Design review of the part built by this model. Coordinates are the model's own, in mm. A direction names the side the tool comes from. Coordinates: 2 decimals unless noted, no trailing zeros. Loops run counter-clockwise (first coordinate to the right, second up) from the corner with the lowest first, then second, coordinate; pieces in that order, holes last. Notation, with made-up numbers: M 14.25,39 L 45.25,39 A26 ccw 45.25,63 Z; hole C 88.25,-7 d11. An arc over 180 degrees is marked long. Answer as a JSON object with one key per item and string values. Group by question number.
1. Consider section B-B (y = 10.9). State the section outline as (x, z) points, then the cut area to 3 significant figures.
2. Machinability: for faces 4 (the flat face through (4, 20.2, 5)), 5 (the flat face through (8, 21, 5)), 6 (the flat face through (16, 0, 1)), which of the approach directions +Z, -Z, +X, -X, +Y, -Y give a long, thin tool a straight path to every point of the face, cutting with its end or side? Answer none if there is none.
3. Draft analysis for pull direction Y (two halves, no side actions). For faces 1 (the flat face through (0, 11, 1)), 2 (the flat face through (16, 21.8, 1)), 3 (the flat face through (4, 1.6, 5)), state which applies: +Y half, -Y half, draft (parallel to the pull), parting line (faces both ways), or undercut.
4. To check wall thickness, follow probe 1 along Y at (x, z) = (18, 0.5); probe 2 along Z at (x, y) = (48.5, 10.5); probe 3 along X at (y, z) = (10.5, 0.75). State the ranges of each line that lie inside material, in increasing order.
5. Consider section D-D (y = 3.5). State the section outline as (x, z) points.
6. Consider section A-A (z = 3). State the section outline as (x, y) points.
7. Insertion check: pin 1 (5 mm diameter, centred on y = 18.5, z = 10, fed in from +X); pin 2 (4 mm diameter, centred on x = 18, y = 10.9, fed in from +Z). Each pin has a flat end and moves straight along its axis. Give the tip position at first contact, or say it passes through.
8. Consider section C-C (x = 42). State the section outline as (y, z) points.
Autodesk Inventor part; units mm, degrees
ref_plane "YZ Plane" through (0, 0, 0) normal (1, 0, 0) x (0, 1, 0)
ref_plane "XZ Plane" through (0, 0, 0) normal (0, 1, 0) x (-1, 0, 0)
ref_plane "XY Plane" through (0, 0, 0) normal (0, 0, 1) x (1, 0, 0)
sketch "Sketch1" plane through (0, 0, 0) normal (0, 0, 1) x (1, 0, 0)
  line L0 (0, 0) -> (50, 0)
  line L1 (50, 0) -> (50, 21.8)
  line L2 (50, 21.8) -> (0, 21.8)
  line L3 (0, 21.8) -> (0, 0)
  circle A0 centre (42, 10.9) radius 1.65
  circle A1 centre (18, 10.9) radius 1.65
  dimension "d0" = 50
  dimension "d1" = 21.8
  dimension "d15" = 3.3
  dimension "d16" = 3.3
  dimension "d17" = 24
  dimension "d18" = 8
  dimension "d19" = 10.9
  dimension "d20" = 10.9
extrude "Extrusion1" add sketch "Sketch1" along normal blind 1.6
sketch "Sketch2" plane through (0, 0, 1.6) normal (0, 0, 1) x (1, 0, 0)
  line L0 (0, 21.8) -> (0, 0)
  line L1 (0, 0) -> (8, 0)
  line L2 (8, 0) -> (8, 1.6)
  line L3 (8, 1.6) -> (0, 1.6)
  line L4 (0, 1.6) -> (0, 0)
  line L5 (50, 21.8) -> (0, 21.8)
  line L6 (0, 21.8) -> (8, 21.8)
  line L7 (8, 21.8) -> (8, 20.2)
  line L8 (8, 20.2) -> (0, 20.2)
  line L9 (0, 20.2) -> (0, 21.8)
  point P0 (0, 20.2)
  dimension "d4" = 8
  dimension "d5" = 1.6
  dimension "d6" = 8
  dimension "d7" = 1.6
extrude "Extrusion2" add sketch "Sketch2" along normal blind 10
sketch "Sketch3" plane through (0, 0, 0) normal (0, -1, 0) x (1, 0, 0)
  circle A0 centre (4, 7.1) radius 1.65
  line L0 (0, 0) -> (0, 11.6)
  line L1 (0, 11.6) -> (8, 11.6)
  line L2 (0, 0) -> (50, 0)
  dimension "d10" = 3.3
  dimension "d11" = 4
  dimension "d21" = 7.1
extrude "Extrusion3" cut sketch "Sketch3" against normal blind 25
fillet "Fillet1" radius 4 4 edges at (8, 0.8, 11.6) (8, 21, 11.6) (0, 0.8, 11.6) (0, 21, 11.6)
properties part number "Base"
Findings below:
{
 "1": {"outline": "M 0,0 L 16.35,0 L 16.35,1.6 L 0,1.6 Z; M 19.65,0 L 40.35,0 L 40.35,1.6 L 19.65,1.6 Z; M 43.65,0 L 50,0 L 50,1.6 L 43.65,1.6 Z", "area": "69.4 mm^2"},
 "2": {"face 4": "+Z, +X, -X", "face 5": "+Z, +X, +Y, -Y", "face 6": "+Z, -Z, +X, -X, -Y"},
 "3": {"face 1": "draft", "face 2": "+Y half", "face 3": "undercut"},
 "4": {"probe 1": "y = 0 to 9.25, 12.55 to 21.8", "probe 2": "z = 0 to 1.6", "probe 3": "x = 0 to 16.4, 19.6 to 40.4, 43.6 to 50"},
 "5": {"outline": "M 0,0 L 50,0 L 50,1.6 L 0,1.6 Z"},
 "6": {"outline": "M 0,0 L 8,0 L 8,1.6 L 0,1.6 Z; M 0,20.2 L 8,20.2 L 8,21.8 L 0,21.8 Z"},
 "7": {"pin 1": "stops at x = 7.96", "pin 2": "stops at z = 1.6"},
 "8": {"outline": "M 0,0 L 9.25,0 L 9.25,1.6 L 0,1.6 Z; M 12.55,0 L 21.8,0 L 21.8,1.6 L 12.55,1.6 Z"}
}
